```python
from build123d import *

# Parameters (mm, degrees)
F1_DEPTH = 38.1
F2_DEPTH = 12.7
F4_DEPTH = 25.4
F6_DEPTH = 101.608358


with BuildPart() as f1:
    # F0 (on Top) → F1 (new body, symmetric)
    with BuildSketch(Plane.XY):
        Polygon((25.4, -50.8), (-25.4, -50.8), (0, -101.6), align=None)
        Polygon((50.8, 0), (-50.8, 0), (-25.4, -50.8), (25.4, -50.8), align=None)
    extrude(amount=F1_DEPTH, both=True)

    # F0 (on Top) → F2 (cut, symmetric)
    with BuildSketch(Plane.XY):
        Polygon((25.4, -50.8), (-25.4, -50.8), (0, -101.6), align=None)
    extrude(amount=F2_DEPTH, both=True, mode=Mode.SUBTRACT)

    # F3 (on face) → F4 (join)
    with BuildSketch(Plane(origin=(0, 0, -38.1), x_dir=(1, 0, 0), z_dir=(0, 0, -1))):
        Polygon((0, 101.6), (-50.8, 0), (50.8, 0), align=None)
        with BuildLine():
            ThreePointArc((-101.6, 12.7), (-97.880256, 3.719744), (-88.9, 0))
            Line((-88.9, 0), (-50.8, 0))
            Line((-50.8, 0), (0, 101.6))
            Line((0, 101.6), (50.8, 0))
            Line((50.8, 0), (88.9, 0))
            ThreePointArc((88.9, 0), (97.880256, 3.719744), (101.6, 12.7))
            Line((101.6, 12.7), (101.6, 31.75))
            Line((101.6, 31.75), (63.5, 31.75))
            Line((63.5, 31.75), (63.5, 69.858358))
            Line((63.5, 69.858358), (101.6, 69.858358))
            Line((101.6, 69.858358), (101.6, 88.908358))
            ThreePointArc((101.6, 88.908358), (97.880256, 97.888614), (88.9, 101.608358))
            Line((88.9, 101.608358), (-88.9, 101.608358))
            ThreePointArc((-88.9, 101.608358), (-97.880256, 97.888614), (-101.6, 88.908358))
            Line((-101.6, 88.908358), (-101.6, 69.858358))
            Line((-101.6, 69.858358), (-63.5, 69.858358))
            Line((-63.5, 69.858358), (-63.5, 31.75))
            Line((-63.5, 31.75), (-101.6, 31.75))
            Line((-101.6, 31.75), (-101.6, 12.7))
        make_face()
    extrude(amount=F4_DEPTH)

    # F5 (on face) → F6 (join, through all)
    with BuildSketch(Plane.XZ.offset(101.608358)):
        Polygon((-31.75, -63.5), (-57.15, -63.5), (-57.15, -88.9), (-31.75, -88.9), (-31.75, -69.85), align=None)
        with BuildLine():
            Line((-25.4, -63.5), (-31.75, -63.5))
            Line((-31.75, -63.5), (-31.75, -69.85))
            ThreePointArc((-31.75, -69.85), (-29.890128, -65.359872), (-25.4, -63.5))
        make_face()
        with BuildLine():
            Line((31.75, -63.5), (25.4, -63.5))
            ThreePointArc((25.4, -63.5), (29.890128, -65.359872), (31.75, -69.85))
            Line((31.75, -69.85), (31.75, -63.5))
        make_face()
        Polygon((31.75, -63.5), (31.75, -69.85), (31.75, -88.9), (57.15, -88.9), (57.15, -63.5), align=None)
    extrude(amount=-F6_DEPTH)


solid = f1.part
```
Check sheet for the modelled part. Datum: model origin and axes. Units: mm. A direction names the side the tool comes from. Give positions to 0.01 mm unless a question says otherwise; leave off trailing zeros. Order: outer loops, then holes, each group sorted by start corner. A loop starts at its lowest first (then second) coordinate and runs counter-clockwise, first axis right, second up. Notation, with made-up numbers: M 76.5,6 L 85.5,6 A29 ccw 85.5,26 Z; hole C 78,70.25 d10. An arc over 180 degrees is marked long. Answer in a Markdown table with one row per item.
1) Thickness scan on L1, parallel to Z at x = -10, y = -58; L2, parallel to Y at x = 82, z = -61; L3, parallel to X at y = -53.5, z = -70.5. Record the ranges inside material, lowest first. Write a range as [from, to].
Filled sheet:
| item | result |
|---|---|
| L1 | z = [-63.5, -12.7], [12.7, 38.1] |
| L2 | y = [-101.61, -69.86], [-31.75, 0] |
| L3 | x = [-57.15, -31.75], [31.75, 57.15] |
2) Cross-section at D-D, the plane y = -65. Enter the section's corners in (x, z).
Filled sheet:
| item | result |
|---|---|
| outline | M -63.5,-63.5 L -57.15,-63.5 L -57.15,-88.9 L -31.75,-88.9 L -31.75,-69.85 A6.35 cw -25.4,-63.5 L 25.4,-63.5 A6.35 cw 31.75,-69.85 L 31.75,-88.9 L 57.15,-88.9 L 57.15,-63.5 L 63.5,-63.5 L 63.5,-38.1 L 18.3,-38.1 L 18.3,-12.7 L -18.3,-12.7 L -18.3,-38.1 L -63.5,-38.1 Z; M -18.3,12.7 L 18.3,12.7 L 18.3,38.1 L -18.3,38.1 Z |
3) Access from +Z, -Z, +X, -X, +Y, -Y to the whole of each face (thin tool, end or side, straight path). Record for faces 5 (the flat face through (0, -70, 12.7)), 6 (the flat face through (-83, -69.858, -51)), 7 (the flat face through (-57.15, -52, -76)).
Filled sheet:
| item | result |
|---|---|
| face 5 | +X, -X, -Y |
| face 6 | +Z, -Z, -X |
| face 7 | -Z, -X, +Y, -Y |
4) Gauge pin test, flat ends, axial feed: P1, Ø5.5, axis at y = -47.5, z = -79, coming from the -X side; P2, Ø4, axis at y = -75, z = 22, coming from the +X side; P3, Ø2, axis at x = 77.5, z = -37, coming from the -Y side; P4, Ø4, axis at x = 68, y = -87, coming from the +Z side. Record the tip position at first contact, or that the pin passes through.
Filled sheet:
| item | result |
|---|---|
| P1 | stops at x = -57.15 |
| P2 | stops at x = 14.3 |
| P3 | passes through |
| P4 | stops at z = -38.1 |
5) Release check for a two-part mould opening along X. For faces 1 (the cylindrical face through (-97.98, -3.82, -50.62)), 2 (the flat face through (30.7, -40.2, 0.5)), 3 (the flat face through (31.75, -52, -79)), 4 (the flat face through (-31.75, -52, -80)) record: +X half, -X half, draft (parallel to the pull), parting line (faces both ways), or undercut.
Filled sheet:
| item | result |
|---|---|
| face 1 | -X half |
| face 2 | +X half |
| face 3 | undercut |
| face 4 | undercut |
6) Cross-section at B-B, the plane x = 2.5. Enter the section's corners in (y, z).
Filled sheet:
| item | result |
|---|---|
| outline | M -101.61,-63.5 L 0,-63.5 L 0,38.1 L -96.6,38.1 L -96.6,12.7 L -50.8,12.7 L -50.8,-12.7 L -96.6,-12.7 L -96.6,-38.1 L -101.61,-38.1 Z |
7) Cross-section at C-C, the plane x = 82.5. Enter the section's corners in (y, z), plus the area to 3 significant figures.
Filled sheet:
| item | result |
|---|---|
| outline | M -101.61,-63.5 L -69.86,-63.5 L -69.86,-38.1 L -101.61,-38.1 Z; M -31.75,-63.5 L 0,-63.5 L 0,-38.1 L -31.75,-38.1 Z |
| area | 1,610 mm2 |
8) Cross-section at A-A, the plane y = -84. Enter the section's corners in (x, z), plus the area to 3 significant figures.
Filled sheet:
| item | result |
|---|---|
| outline | M -101.6,-63.5 L -57.15,-63.5 L -57.15,-88.9 L -31.75,-88.9 L -31.75,-69.85 A6.35 cw -25.4,-63.5 L 25.4,-63.5 A6.35 cw 31.75,-69.85 L 31.75,-88.9 L 57.15,-88.9 L 57.15,-63.5 L 101.6,-63.5 L 101.6,-38.1 L 8.8,-38.1 L 8.8,-12.7 L -8.8,-12.7 L -8.8,-38.1 L -101.6,-38.1 Z; M -8.8,12.7 L 8.8,12.7 L 8.8,38.1 L -8.8,38.1 Z |
| area | 7,360 mm2 |
